Read the model definition and answer for the solid it produces. Units are mm, in the model's axes. Face numbers are marked on the shaded views. A direction names the side the tool comes from. Give positions to 0.01 mm unless a question says otherwise; leave off trailing zeros. Order: outer loops, then holes, each group sorted by start corner. A loop starts at its lowest first (then second) coordinate and runs counter-clockwise, first axis right, second up. Notation, with made-up numbers: (-35, 6) - (-11, 6) arc R5 ccw to (-11, 12) - close; hole circle Ø7 at (-19.75, 42). An arc over 180 degrees is marked (long way). Use a Markdown table: item, result. Add a question column.
1. Which of the six approach directions +Z, -Z, +X, -X, +Y, -Y give full straight-line access (tool end or side, diameter ignored) to the marked faces 1 and 2?
2. A cutting plane is placed at B-B on z = -1.65. Determine the outline of the cut face in (x, y).
3. For a pull along X with two mould halves and no side action, classify the marked faces 3, 4 and 5 as released by +X, released by -X, zero draft, split by the parting line, or undercut.
4. A cutting plane is placed at A-A on x = 0. Determine the outline of the cut face in (y, z), and give its area (3 significant figures).
5. A cutting plane is placed at D-D on y = 13.5. Determine the outline of the cut face in (x, z), and give its area (3 significant figures).
6. Flat-ended cylindrical pins translate along their axes: P1, Ø2.5, axis at x = 0, y = 30, coming from the -Z side; P2, Ø1.5, axis at x = 1, z = -1, coming from the +Y side; P3, Ø2, axis at x = -2.5, z = 1, coming from the +Y side; P4, Ø1.5, axis at y = 16.5, z = -1, coming from the -X side. Find the tip coordinate at first contact, or state that the pin passes through.
7. Consider L1, parallel to Y at x = 0, z = -1.7; L2, parallel to Y at x = -1, z = 0.8; L3, parallel to Y at x = 0, z = 1.8. Determine where each line is inside the solid, lowest interval first.
8. A cutting plane is placed at C-C on z = 2.35. Determine the outline of the cut face in (x, y), and give its area (3 significant figures).
```python
from build123d import *

# Parameters (mm, degrees)
SKETCH2_R               = 1.5
BOSS_EXTRUDE1_DEPTH     = 3
CUT_EXTRUDE1_DEPTH      = 1
CUT_EXTRUDE1_DEPTH_BACK = 4


with BuildPart() as part:
    # Sketch2 → Boss-Extrude1 (new body, symmetric)
    with BuildSketch(Plane.XY):
        with BuildLine():
            Line((-4.99722145, 0.166666667), (-3.99777716, 30.133333333))
            ThreePointArc((-3.99777716, 30.133333333), (0, 34), (3.99777716, 30.133333333))
            Line((3.99777716, 30.133333333), (4.99722145, 0.166666667))
            ThreePointArc((4.99722145, 0.166666667), (0, -5), (-4.99722145, 0.166666667))
        make_face()
        with Locations((0, 30)):
            Circle(SKETCH2_R, mode=Mode.SUBTRACT)
    extrude(amount=BOSS_EXTRUDE1_DEPTH, both=True)

    # Sketch1 → Cut-Extrude1 (cut, two sides)
    with BuildSketch(Plane.XY) as cut_extrude1_sk:
        with BuildLine():
            Line((-1.99119154, 16.1875), (-3.484585195, 0.328125))
            ThreePointArc((-3.484585195, 0.328125), (0, -3.5), (3.484585195, 0.328125))
            Line((3.484585195, 0.328125), (1.99119154, 16.1875))
            ThreePointArc((1.99119154, 16.1875), (0, 18), (-1.99119154, 16.1875))
        make_face()
    extrude(amount=CUT_EXTRUDE1_DEPTH, mode=Mode.SUBTRACT)
    extrude(cut_extrude1_sk.sketch, amount=-CUT_EXTRUDE1_DEPTH_BACK, mode=Mode.SUBTRACT)


solid = part.part
```
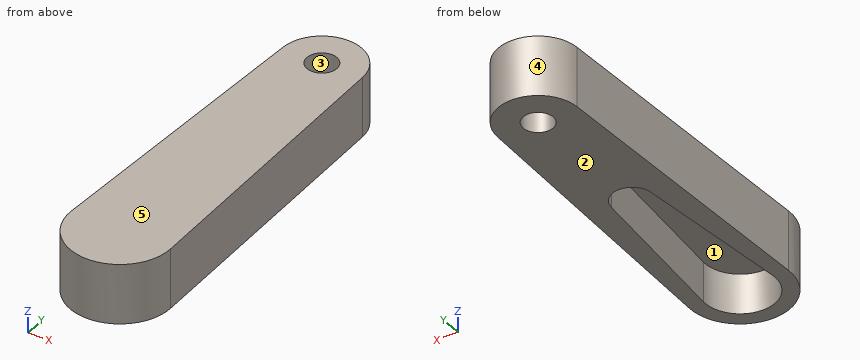
Output values:
| question | item | result |
|---|---|---|
| 1 | face 1 | -Z |
| 1 | face 2 | -Z, +X, -X, +Y, -Y |
| 2 | outline | (-5, 0.17) arc R5 ccw (long way) to (5, 0.17) - (4, 30.13) arc R4 ccw to (-4, 30.13) - close; hole (-3.48, 0.33) arc R3.5 ccw (long way) to (3.48, 0.33) - (1.99, 16.19) arc R2 ccw to (-1.99, 16.19) - close; hole circle Ø3 at (0, 30) |
| 3 | face 3 | undercut |
| 3 | face 4 | split by the parting line |
| 3 | face 5 | zero draft |
| 4 | outline | (-5, -3) - (-3.5, -3) - (-3.5, 1) - (18, 1) - (18, -3) - (28.5, -3) - (28.5, 3) - (-5, 3) - close; (31.5, -3) - (34, -3) - (34, 3) - (31.5, 3) - close |
| 4 | area | 130 mm² |
| 5 | outline | (-4.55, -3) - (-2.24, -3) - (-2.24, 1) - (2.24, 1) - (2.24, -3) - (4.55, -3) - (4.55, 3) - (-4.55, 3) - close |
| 5 | area | 36.7 mm² |
| 6 | P1 | through |
| 6 | P2 | y = 33.99 |
| 6 | P3 | y = 33.71 |
| 6 | P4 | x = -4.48 |
| 7 | L1 | -5 to -3.5, 18 to 28.5, 31.5 to 34 |
| 7 | L2 | -4.9 to -3.35, 17.73 to 28.88, 31.12 to 33.87 |
| 7 | L3 | -5 to 28.5, 31.5 to 34 |
| 8 | outline | (-5, 0.17) arc R5 ccw (long way) to (5, 0.17) - (4, 30.13) arc R4 ccw to (-4, 30.13) - close; hole circle Ø3 at (0, 30) |
| 8 | area | 327 mm² |
